Verification items for this drawing (mm, ordinates from the low corner). A direction names the side the tool comes from. Coordinates: 2 decimals unless noted, no trailing zeros. Order: outer loops, then holes, each group sorted by start corner. A loop starts at its lowest first (then second) coordinate and runs counter-clockwise, first axis right, second up.
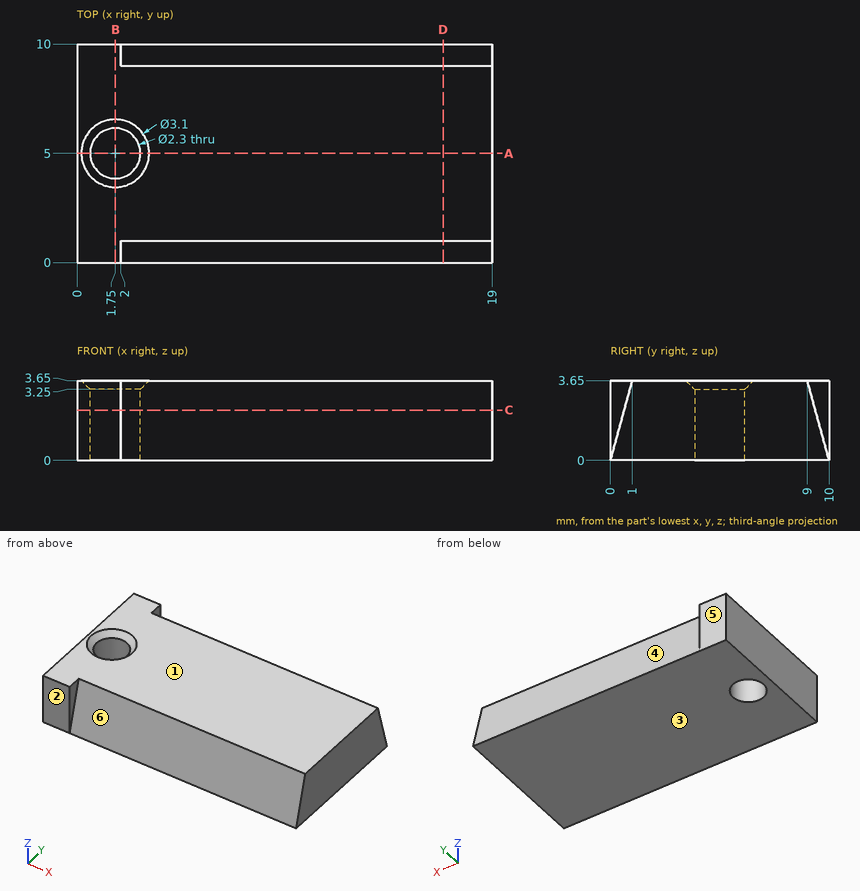
(1) Release check for a two-part mould opening along Z. For the marked faces 1, 2 and 3 record: +Z half, -Z half, draft (parallel to the pull), parting line (faces both ways), or undercut.
Filled in:
face 1: +Z half
face 2: draft
face 3: -Z half
(2) Thickness scan on probe 1 along X at (y, z) = (5, 2.95); probe 2 along X at (y, z) = (4, 2.9); probe 3 along Y at (x, z) = (8.5, 2.45). Record the ranges inside material, lowest first.
Filled in:
probe 1: x = 0 to 0.6, 2.9 to 19
probe 2: x = 0 to 1.18, 2.32 to 19
probe 3: y = 0.67 to 9.33
(3) Cross-section at B-B (x = 1.75). Enter the section's corners in (y, z), and give its area (3 significant figures).
Filled in:
outline: (0, 0) - (3.85, 0) - (3.85, 3.25) - (3.45, 3.65) - (0, 3.65) - close; (6.15, 0) - (10, 0) - (10, 3.65) - (6.55, 3.65) - (6.15, 3.25) - close
area: 27.9 mm2
(4) Cross-section at C-C (z = 2.3). Enter the section's corners in (x, y).
Filled in:
outline: (0, 0) - (2, 0) - (2, 0.63) - (19, 0.63) - (19, 9.37) - (2, 9.37) - (2, 10) - (0, 10) - close; hole circle Ø2.3 at (1.75, 5)
(5) Cross-section at D-D (x = 16.75). Enter the section's corners in (y, z), and give its area (4 significant figures).
Filled in:
outline: (0, 0) - (10, 0) - (9, 3.65) - (1, 3.65) - close
area: 32.85 mm2
(6) Tool access check on the marked faces 4, 5 and 6. Record the directions out of +Z, -Z, +X, -X, +Y, -Y that give a thin tool (end or side, any length) a straight path to the whole face; none if there is none.
Filled in:
face 4: +Z, +X, +Y
face 5: +Z, -Z, +X, -X, +Y
face 6: +Z, +X, -Y
(7) Cross-section at A-A (y = 5). Enter the section's corners in (x, z), and give its area (3 significant figures).
Filled in:
outline: (0, 0) - (0.6, 0) - (0.6, 3.25) - (0.2, 3.65) - (0, 3.65) - close; (2.9, 0) - (19, 0) - (19, 3.65) - (3.3, 3.65) - (2.9, 3.25) - close
area: 60.8 mm2
(8) Go/stop test with a flat-tipped pin: P1, Ø2, axis at x = 1.75, y = 5, coming from the +Z side. Record where the tip stops, or that it passes through.
Filled in:
P1: passes through
